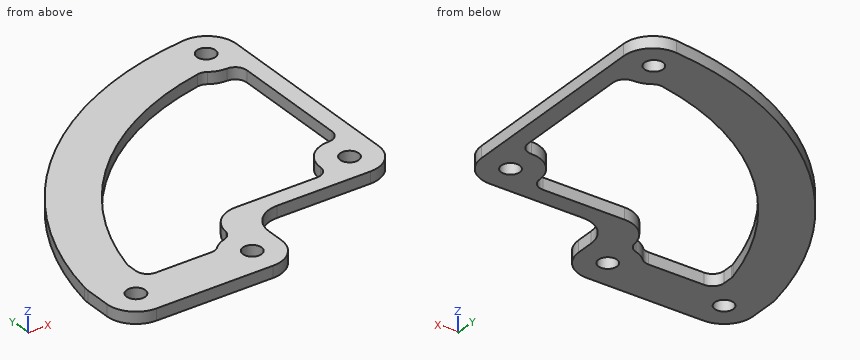
```python
from build123d import *

# Parameters (mm, degrees)
SKETCH_1_R      = 1.6
EXTRUDE_1_DEPTH = 2
FILLET_1_R      = 5
FILLET_2_R      = 2


with BuildPart() as part:
    # ｽｹｯﾁ1 → ﾎﾞｽ - 押し出し1 (new body)
    with BuildSketch(Plane.XY):
        with BuildLine():
            Line((-30, 10), (-30, 0))
            Line((-30, 0), (0, 0))
            Line((0, 0), (0, 13))
            Line((0, 13), (26, 13))
            Line((26, 13), (26, 57.5))
            ThreePointArc((26, 57.5), (-10.715970639, 44.025670649), (-30, 10))
        make_face()
        with Locations((-25, 5)):
            Circle(SKETCH_1_R, mode=Mode.SUBTRACT)
        with Locations((-5, 5)):
            Circle(SKETCH_1_R, mode=Mode.SUBTRACT)
        with Locations((21, 18)):
            Circle(SKETCH_1_R, mode=Mode.SUBTRACT)
        with Locations((21, 52.5)):
            Circle(SKETCH_1_R, mode=Mode.SUBTRACT)
        with BuildLine():
            Line((-5, 11), (-5, 10))
            ThreePointArc((-5, 10), (-7.236067977, 9.472135955), (-9, 8))
            Line((-9, 8), (-21.442485956, 8))
            Line((-21.442485956, 8), (-21.442485956, 12))
            ThreePointArc((-21.442485956, 12), (-7.409474557, 36.255609967), (17.657876922, 48.781100521))
            ThreePointArc((17.657876922, 48.781100521), (19.210376771, 47.83124763), (21, 47.5))
            Line((21, 47.5), (23, 47.5))
            Line((23, 47.5), (23, 23))
            Line((23, 23), (21, 23))
            ThreePointArc((21, 23), (17.464466094, 21.535533906), (16, 18))
            Line((16, 18), (16, 16))
            Line((16, 16), (0, 16))
            ThreePointArc((0, 16), (-3.535533906, 14.535533906), (-5, 11))
        make_face(mode=Mode.SUBTRACT)
    extrude(amount=EXTRUDE_1_DEPTH)

    # ﾌｨﾚｯﾄ1
    fillet_1_edges = [part.edges().sort_by_distance(p)[0] for p in [
        (26, 57.5, 1),
        (26, 13, 1),
        (0, 13, 1),
        (0, 0, 1),
        (-30, 0, 1),
        (-30, 10, 1),
    ]]
    fillet(fillet_1_edges, radius=FILLET_1_R)

    # ﾌｨﾚｯﾄ2
    fillet_2_edges = [part.edges().sort_by_distance(p)[0] for p in [
        (17.657876922, 48.781100521, 1),
        (23, 47.5, 1),
        (16, 16, 1),
        (23, 23, 1),
        (-5, 10, 1),
        (-9, 8, 1),
        (-21.442485956, 8, 1),
        (-21.442485956, 12, 1),
    ]]
    fillet(fillet_2_edges, radius=FILLET_2_R - 0.0001)  # a hair under: the kernel refuses the full size


solid = part.part
```
For this review, take the finished solid that the model builds, in its own axes (mm). Give positions to 0.01 mm unless a question says otherwise; leave off trailing zeros. Order: outer loops, then holes, each group sorted by start corner. A loop starts at its lowest first (then second) coordinate and runs counter-clockwise, first axis right, second up.
1) Wall thickness on line 1 (X direction, y = 17, z = 1.5); line 2 (Y direction, x = 21, z = 0.7); line 3 (X direction, y = 30, z = 0.5): over which ranges is each line inside the solid? List them lowest first.
2) Take a section at A-A (x = 1). Give the boundary of the cut face in (y, z), then the cut area to 3 significant figures.
3) Take a section at B-B (y = 38). Give the boundary of the cut face in (x, z), then the cut area to 3 significant figures.
4) Insertion check: pin 1 (1 mm diameter, centred on x = -21.5, z = 1.5, fed in from +Y); pin 2 (1 mm diameter, centred on x = 11, z = 1.5, fed in from -Y); pin 3 (1 mm diameter, centred on y = 39, z = 1, fed in from -X). Each pin has a flat end and moves straight along its axis. Give the tip position at first contact, or say it passes through.
5) Take a section at C-C (z = 1.2). State how many separate pieces and enclosed holes the cut face has, then the cut area to 3 significant figures.
Derived:
1. line 1: x = -28.38 to -19.97, 15.73 to 19.75, 22.25 to 25.9
1. line 2: y = 13 to 16.4, 19.6 to 23, 47.5 to 50.9, 54.1 to 57.26
1. line 3: x = -22.64 to -13.01, 23 to 26
2. outline: (11, 0) - (16, 0) - (16, 2) - (11, 2) - close; (42.6, 0) - (51.7, 0) - (51.7, 2) - (42.6, 2) - close
2. area: 28.2 mm2
3. outline: (-16.82, 0) - (-5.45, 0) - (-5.45, 2) - (-16.82, 2) - close; (23, 0) - (26, 0) - (26, 2) - (23, 2) - close
3. area: 28.7 mm2
4. pin 1: stops at y = 32.56
4. pin 2: stops at y = 13
4. pin 3: stops at x = -16.38
5. separate pieces: 1
5. enclosed holes: 5
5. area: 1,070 mm2
